```python
from build123d import *

# Parameters (mm, degrees)
SKETCH1_W                = 20
SKETCH1_H                = 20
SKETCH1_R                = 5.3
BOSS_EXTRUDE1_DEPTH      = 10
SKETCH2_W                = 20
SKETCH2_H                = 20
BOSS_EXTRUDE2_DEPTH      = 5
BOSS_EXTRUDE6_DEPTH      = 20
BOSS_EXTRUDE6_DEPTH_BACK = 5
SKETCH9_W                = 20
SKETCH9_H                = 20
F_6_0_6_DIAMETER_HOLE3_D = 6
FILLET3_R                = 10
FILLET6_R                = 3


with BuildPart() as part:
    # Sketch1 → Boss-Extrude1 (new body)
    with BuildSketch(Plane(origin=(0, 0, 0), x_dir=(0, 0, -1), z_dir=(1, 0, 0))):
        Rectangle(SKETCH1_W, SKETCH1_H)
        Circle(SKETCH1_R, mode=Mode.SUBTRACT)
    extrude(amount=BOSS_EXTRUDE1_DEPTH)

    # Sketch2 → Boss-Extrude2 (add)
    with BuildSketch(Plane(origin=(10, 0, 0), x_dir=(0, 0, -1), z_dir=(1, 0, 0))):
        Rectangle(SKETCH2_W, SKETCH2_H)
    extrude(amount=BOSS_EXTRUDE2_DEPTH)

    # Sketch9 → Boss-Extrude6 (add, two sides: drawn at the far end of the back side and taken through both)
    with BuildSketch(Plane(origin=(15, 0, 0), x_dir=(0, 0, -1), z_dir=(1, 0, 0)).offset(-BOSS_EXTRUDE6_DEPTH_BACK)):
        Rectangle(SKETCH9_W, SKETCH9_H)
    extrude(amount=BOSS_EXTRUDE6_DEPTH + BOSS_EXTRUDE6_DEPTH_BACK)

    # Ø6.0 (6) Diameter Hole3 (through all)
    with Locations(Plane(origin=(25, 10, 0), x_dir=(0, 0, 1), z_dir=(0, 1, 0))):
        with Locations((0, 0)):
            Hole(F_6_0_6_DIAMETER_HOLE3_D / 2)

    # Fillet3
    fillet3_edges = [part.edges().sort_by_distance(p)[0] for p in [
        (35, 0, -10),
        (35, 0, 10),
    ]]
    fillet(fillet3_edges, radius=FILLET3_R - 0.0001)  # a hair under: the kernel refuses the full size

    # Fillet6
    fillet6_edges = [part.edges().sort_by_distance(p)[0] for p in [
        (12.50005, -10, -10),
        (12.50005, -10, 10),
        (32.071097101, -10, -7.071097101),
        (32.071097101, -10, 7.071097101),
        (12.50005, 10, 10),
        (12.50005, 10, -10),
        (32.071097101, 10, -7.071097101),
        (32.071097101, 10, 7.071097101),
    ]]
    fillet(fillet6_edges, radius=FILLET6_R)


solid = part.part
```
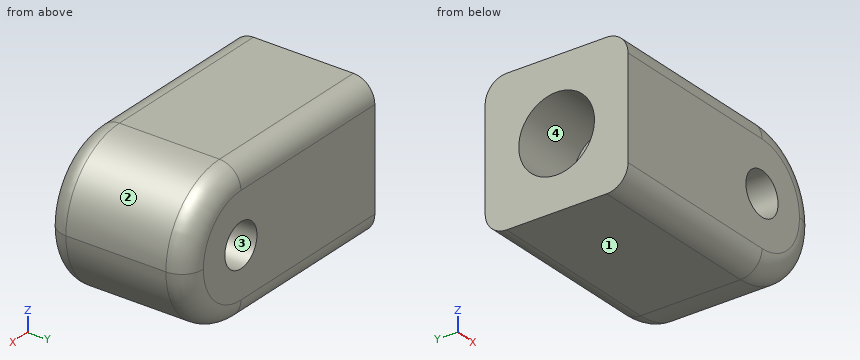
Here's how the part is built. I have some questions about the finished solid (model axes, mm). Face numbers are marked on the shaded views. Coordinates: 2 decimals unless noted, no trailing zeros. Order: outer loops, then holes, each group sorted by start corner. A loop starts at its lowest first (then second) coordinate and runs counter-clockwise, first axis right, second up. Notation, with made-up numbers: M -20,41.25 L -10,41.25 A14 ccw -10,67.25 Z; hole C 58.5,11.25 d10. An arc over 180 degrees is marked long. Answer as a JSON object with one key per item and string values. Group by question number.
(1) Suppose I cut it at C-C, the plane x = 23.5. Please give me the cut outline in (y, z), then the cut area to 3 significant figures.
(2) For pin 1 (6.5 mm diameter, centred on y = 0, z = 0, fed in from -X); pin 2 (2 mm diameter, centred on x = 27.5, y = 5, fed in from +Z), each with a flat end and sliding along its axis, tell me the tip position at first contact or that it passes through.
(3) I need wall thicknesses on probe 1 along Y at (x, z) = (4, 0); probe 2 along X at (y, z) = (0, 0); probe 3 along Z at (x, y) = (6, 0.5). Which ranges of each line are inside material? Lowest first, please.
(4) If we mould it in two halves opening along Z, with no side actions, what happens to the marked faces 1, 2, 3 and 4? For each: released by +Z, released by -Z, zero draft, split by the parting line, or undercut.
(5) Suppose I cut it at A-A, the plane x = 4. Please give me the cut outline in (y, z), then the cut area to 3 significant figures.
Values found:
{
 "1": {"outline": "M -10,-7 A3 ccw -7,-10 L 7,-10 A3 ccw 10,-7 L 10,-2.6 L -10,-2.6 Z; M -10,2.6 L 10,2.6 L 10,7 A3 ccw 7,10 L -7,10 A3 ccw -10,7 Z", "area": "288 mm^2"},
 "2": {"pin 1": "stops at x = 10", "pin 2": "stops at z = 9.89"},
 "3": {"probe 1": "y = -10 to -5.3, 5.3 to 10", "probe 2": "x = 10 to 22, 28 to 35", "probe 3": "z = -10 to -5.28, 5.28 to 10"},
 "4": {"face 1": "released by -Z", "face 2": "released by +Z", "face 3": "undercut", "face 4": "undercut"},
 "5": {"outline": "M -10,-7 A3 ccw -7,-10 L 7,-10 A3 ccw 10,-7 L 10,7 A3 ccw 7,10 L -7,10 A3 ccw -10,7 Z; hole C 0,0 d10.6", "area": "304 mm^2"}
}
